For this review, use the dimensioned drawing (mm, ordinates from the lowest corner) and the shaded views. A direction names the side the tool comes from. Coordinates: 2 decimals unless noted, no trailing zeros. Write each loop counter-clockwise with the first axis right and the second up, starting at its lowest first coordinate (ties: lowest second). Pieces come first, ordered by that corner, then holes. Notation, with made-up numbers: M 70,-18 L 107,-18 A6 cw 107,-14 Z; hole C 22.5,16 d10. An arc over 180 degrees is marked long. One line per question, with ' | ' between items.
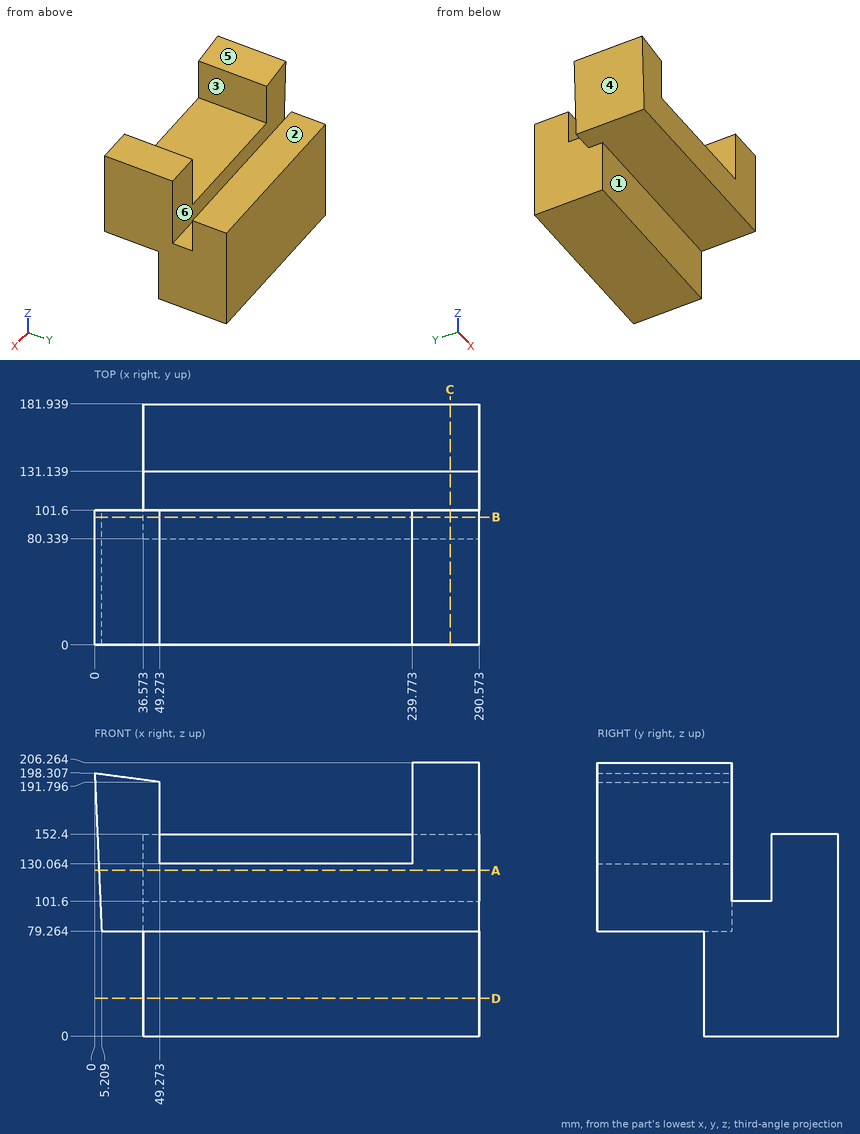
1. Insertion check: pin 1 Ø2 at (x, y) = (220.5, 137.5) entering from +Z; pin 2 Ø3 at (x, y) = (193.5, 64.5) entering from -Z. Each pin has a flat end and moves straight along its axis. Give the tip position at first contact, or say it passes through.
Answer sheet:
pin 1: z = 152.4 | pin 2: z = 79.26
2. Draft analysis for pull direction X (two halves, no side actions). For the marked faces 4, 5 and 6, state which applies: pulls with the +X half, pulls with the -X half, needs draft (parallel to the pull), parting line crosses it, or undercut.
Answer sheet:
face 4: pulls with the -X half | face 5: undercut | face 6: needs draft
3. Take a section at C-C (x = 268.5). Write out the cut boundary in (y, z), then the cut area to 3 significant figures.
Answer sheet:
outline: M 0,79.26 L 80.34,79.26 L 80.34,0 L 181.94,0 L 181.94,152.4 L 131.14,152.4 L 131.14,101.6 L 101.6,101.6 L 101.6,206.26 L 0,206.26 Z | area: 25,300 mm^2
4. To check wall thickness, follow line 1 along Y through (x, z) = (186, 118); line 2 along Z through (x, y) = (53, 52.5); line 3 along X through (y, z) = (153, 52). State the ranges of each line that lie inside material, in increasing order. Write a range as [from, to].
Answer sheet:
line 1: [0, 101.6], [131.14, 181.94] | line 2: [79.26, 130.06] | line 3: [36.57, 290.57]
5. Tool access review of the marked faces 1, 2 and 3: name each direction out of +Z, -Z, +X, -X, +Y, -Y from which nothing blocks a thin tool from reaching the whole face with its end or side.
Answer sheet:
face 1: -Z, +X, -X, -Y | face 2: +Z, +X, -X, +Y | face 3: +Z, -Y
6. Take a section at B-B (y = 96.5). Write out the cut boundary in (x, z).
Answer sheet:
outline: M 0,198.31 L 5.21,79.26 L 36.57,79.26 L 36.57,0 L 290.57,0 L 290.57,206.26 L 239.77,206.26 L 239.77,130.06 L 49.27,130.06 L 49.27,191.8 Z
7. Take a section at D-D (z = 28.5). Write out the cut boundary in (x, y).
Answer sheet:
outline: M 36.57,80.34 L 290.57,80.34 L 290.57,181.94 L 36.57,181.94 Z
8. Take a section at A-A (z = 125). Write out the cut boundary in (x, y), then the cut area to 3 significant figures.
Answer sheet:
outline: M 3.21,0 L 290.57,0 L 290.57,101.6 L 3.21,101.6 Z; M 36.57,131.14 L 290.57,131.14 L 290.57,181.94 L 36.57,181.94 Z | area: 42,100 mm^2
